Autodesk Inventor part; units mm, degrees
ref_plane "YZ Plane" through (0, 0, 0) normal (1, 0, 0) x (0, 1, 0)
ref_plane "XZ Plane" through (0, 0, 0) normal (0, 1, 0) x (-1, 0, 0)
ref_plane "XY Plane" through (0, 0, 0) normal (0, 0, 1) x (1, 0, 0)
sketch "スケッチ1" plane through (0, 0, 0) normal (0, 1, 0) x (-1, 0, 0)
  line L0 (0, -13.02) -> (0, 13.02)
  line L1 (-13.2, 0) -> (16.2, 0)
  line L2 (0, -4.7) -> (-9, -6.5)
  line L3 (-9, -6.5) -> (-9, 6.5)
  line L4 (-9, 6.5) -> (0, 4.7)
  line L5 (0, -9.3) -> (0, -4.7)
  line L6 (0, 4.7) -> (0, 9.3)
  line L7 (2.4, -1.7725) -> (-6.6, -3.5725)
  line L8 (-6.6, -3.5725) -> (-6.6, 3.5725)
  line L9 (-6.6, 3.5725) -> (2.4, 1.7725)
  line L10 (2.4, -6.9) -> (2.4, -1.7725)
  line L11 (2.4, 1.7725) -> (2.4, 6.9)
  line L12 (2.4, -6.9) -> (0, -9.3)
  line L13 (2.4, 6.9) -> (0, 9.3)
  line L14 (12, -6.9) -> (12, 6.9)
  line L15 (12, 6.9) -> (0, 9.3)
  line L16 (12, -6.9) -> (0, -9.3)
  point P0 (0, 0)
  point P1 (0, 9.3)
  point P2 (0, -9.3)
  dimension "d2" = 9
  dimension "d3" = 13
  dimension "d5" = 9.4
  dimension "d13" = 2.4
  dimension "d14" = 2.4
  dimension "d15" = 2.4
  dimension "d24" = 2.4
  dimension "d63" = 2.4
  dimension "d64" = 18.6
  dimension "d65" = 12
  dimension "d74" = 18.6
  dimension "d75" = 2.4
extrude "押し出し2" add sketch "スケッチ1" along normal blind 3.2 and the other way blind 5.2 contours L0 L7 L10 L12 | L2 L3 L1 L8 L7 L0 | L3 L4 L0 L9 L8 L1 | L0 L13 L11 L9
extrude "押し出し1" add sketch "スケッチ1" against normal blind 2
chamfer "面取り4" distance 0.8 angle 45 2 edges at (9, -1, 6.5) (9, -1, -6.5)
chamfer "面取り5" distance 0.8 angle 45 14 edges at (2.1, 0, -2.6725) (6.6, 0, 0) (-2.4, 0, -4.3362) (2.1, 0, 2.6725) (-2.4, 0, 4.3362) (-1.2, 0, 8.1) (-1.2, 0, -8.1) (-1.2, -2, 8.1) (-2.4, -2, 4.3362) (2.1, -2, 2.6725) (6.6, -2, 0) (2.1, -2, -2.6725) (-2.4, -2, -4.3362) (-1.2, -2, -8.1)
equation "\"d2\" = JointMH"
equation "\"d3\" = JointMW1 - 2 * cp"
equation "\"d5\" = JointMW2 - 2 * cp"
equation "\"d13\" = InnerWall"
equation "\"d14\" = InnerWall"
equation "\"d15\" = InnerWall"
equation "\"d24\" = InnerWall"
equation "\"rib\" = 0.5"
equation "\"gap\" = 0.2"
properties part number "StraightRais-215" material "ABS プラスチック"
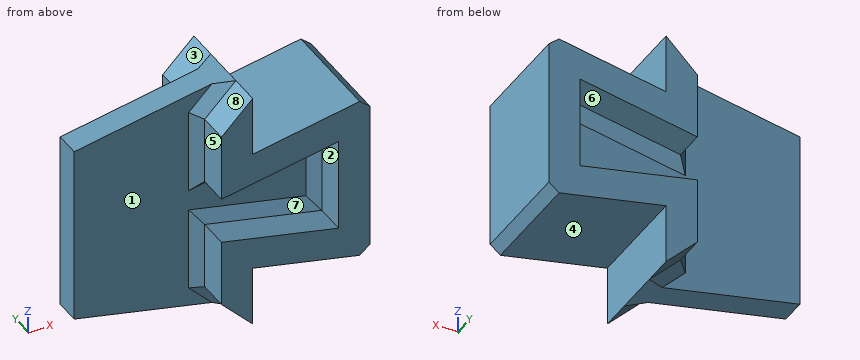
Source: CAD feature listing. Evaluate the final solid. Frame: model axes, mm. Face numbers are marked on the shaded views. A direction names the side the tool comes from. Round coordinates to 2 decimals unless told otherwise and drop trailing zeros. Order: outer loops, then holes, each group sorted by start corner. A loop starts at its lowest first (then second) coordinate and runs counter-clockwise, first axis right, second up. Notation, with made-up numbers: (-20, 13.5) -> (30, 13.5) arc R30 ccw to (30, 45.5) -> close; hole circle Ø2 at (18.5, 21.25). An arc over 180 degrees is marked (long way). One line per item, written item: value. Start each with the question number.
Q1. Section query A-A (z = 5). Return the cut outline in (x, y), plus the area to 3 significant figures.
Q2. Pin query (flat end, axial travel): pin 1 (2.5 mm diameter, centred on y = -1, z = -8, fed in from +X); pin 2 (1.2 mm diameter, centred on y = 2.5, z = 4.5, fed in from -X); pin 3 (1 mm diameter, centred on x = 1.5, y = -0.5, fed in from -Z); pin 4 (2 mm diameter, centred on x = -8.5, y = 1.5, fed in from -Z). Return the tip coordinate at first contact, or that it passes through.
Q3. Section query C-C (z = -0.25). Return the cut outline in (x, y).
Q4. Material intervals for probe 1 along X at (y, z) = (1.25, -0.5); probe 2 along X at (y, z) = (1.25, -6.5); probe 3 along Y at (x, z) = (5.75, -0.25), sorted ascending.
Q5. Section query B-B (y = 2). Return the cut outline in (x, z), plus the area to 3 significant figures.
Q6. Access query for the marked faces 5, 6, 7 and 8. Directions: +Z, -Z, +X, -X, +Y, -Y. A direction counts if a zero-diameter tool reaches every point of the face in a straight line with its end or side. Return the directions, or none.
Q7. Draft query along Z for the marked faces 1, 2, 3 and 4. Return one class per face: pulls with the +Z half, pulls with the -Z half, needs draft (parallel to the pull), parting line crosses it, or undercut.
Q8. Section query D-D (x = -1). Return the cut outline in (y, z), plus the area to 3 significant figures.
Findings below:
1. outline: (-12, -2) -> (-3.2, -2) -> (-2.4, -2.8) -> (-2.4, -5.2) -> (0, -5.2) -> (0, 3.2) -> (-2.4, 3.2) -> (-2.4, 0.8) -> (-3.2, 0) -> (-12, 0) -> close; (1.5, -5.2) -> (9, -5.2) -> (9, 3.2) -> (1.5, 3.2) -> close
1. area: 103 mm²
2. pin 1: x = 0
2. pin 2: x = -2.4
2. pin 3: z = -5.1
2. pin 4: through
3. outline: (-12, -2) -> (5.8, -2) -> (6.6, -2.8) -> (6.6, -5.2) -> (9, -5.2) -> (9, 3.2) -> (6.6, 3.2) -> (6.6, 0.8) -> (5.8, 0) -> (-12, 0) -> close
4. probe 1: 6.6 to 9
4. probe 2: -2.4 to 0
4. probe 3: -2 to 0
5. outline: (-2.4, -6.9) -> (0, -9.3) -> (0, -4.7) -> (8.22, -6.34) -> (9, -5.7) -> (9, 5.7) -> (8.22, 6.34) -> (0, 4.7) -> (0, 9.3) -> (-2.4, 6.9) -> (-2.4, 1.77) -> (6.6, 3.57) -> (6.6, -3.57) -> (-2.4, -1.77) -> close
5. area: 90.9 mm²
6. face 5: +Z, -Z, -X, -Y
6. face 6: +Y
6. face 7: -Y
6. face 8: +Z, -X, -Y
7. face 1: undercut
7. face 2: undercut
7. face 3: pulls with the +Z half
7. face 4: pulls with the -Z half
8. outline: (-5.2, -8.3) -> (-2.8, -8.3) -> (-2.23, -9.1) -> (0.23, -9.1) -> (0.8, -8.3) -> (3.2, -8.3) -> (3.2, -2.05) -> (0.8, -2.05) -> (0, -1.24) -> (0, 1.24) -> (0.8, 2.05) -> (3.2, 2.05) -> (3.2, 8.3) -> (0.8, 8.3) -> (0.23, 9.1) -> (-2.23, 9.1) -> (-2.8, 8.3) -> (-5.2, 8.3) -> (-5.2, 2.05) -> (-2.8, 2.05) -> (-2, 1.24) -> (-2, -1.24) -> (-2.8, -2.05) -> (-5.2, -2.05) -> close
8. area: 119 mm²
